```python
from build123d import *

# Parameters (mm, degrees)
IMPORTED_BODY_4_1_OUTLINE_W = 30
IMPORTED_BODY_4_1_OUTLINE_H = 14
IMPORTED_BODY_4_1_DEPTH     = 3
SKETCH_1_R                  = 3.5
SKETCH_1_R_2                = 2
SKETCH_1_R_3                = 6
CUT_EXTRUDE_1_DEPTH         = 3


# Read off the part's stored shape, not the designer's step: 基体零件-零件4-1
with BuildPart() as part:
    # 基体零件-零件4-1 outline → 基体零件-零件4-1 (new body)
    with BuildSketch(Plane.XY):
        Polygon((110, 31), (0, 31), (0, 20), (-3, 20), (-3, 10), (0, 10), (0, 0), (20, 0), (20, -3), (30, -3), (30, 0), (70, 0), (70, -3), (80, -3), (80, 0), (120, 0), (120, -3), (130, -3), (130, 0), (170, 0), (170, -3), (180, -3), (180, 0), (220, 0), (220, -3), (230, -3), (230, 0), (270, 0), (270, -3), (280, -3), (280, 0), (300, 0), (300, 10), (303, 10), (303, 20), (300, 20), (300, 31), (140, 31), (140, 23), (110, 23), align=None)
        with Locations((125, 13)):
            Rectangle(IMPORTED_BODY_4_1_OUTLINE_W, IMPORTED_BODY_4_1_OUTLINE_H, mode=Mode.SUBTRACT)
    extrude(amount=IMPORTED_BODY_4_1_DEPTH)

    # 草图1 → 切除-拉伸1 (cut)
    with BuildSketch(Plane(origin=(0, 0, 0), x_dir=(-1, 0, 0), z_dir=(0, 0, -1))):
        with Locations(Location((-147.5, 10, 0), (0, 0, 180))):
            Circle(SKETCH_1_R)
        with Locations(Location((-95, 3.5, 0), (0, 0, 180))):
            Circle(SKETCH_1_R_2)
        with Locations((-155.5, 27.5)):
            Circle(SKETCH_1_R_3)
    extrude(amount=-CUT_EXTRUDE_1_DEPTH, mode=Mode.SUBTRACT)


solid = part.part
```
Input: part model. Units: mm. Frame: model coordinates. Give positions to 0.01 mm unless a question says otherwise; leave off trailing zeros. Order: outer loops, then holes, each group sorted by start corner. A loop starts at its lowest first (then second) coordinate and runs counter-clockwise, first axis right, second up. Notation, with made-up numbers: M 88,88 L 135,88 A18 cw 135,110 Z; hole C 23.5,54 d5. An arc over 180 degrees is marked long. Return JSON: item names as keys, results as strings.
Item 1: Pull-direction query (X, two-part tool) for faces 1 (the flat face through (148, 14, 0)), 2 (the cylindrical face through (155.684, 21.503, 1.479)), 3 (the cylindrical face through (150.84, 8.95, 1.48)); classes: +X half, -X half, draft (parallel to the pull), parting line (faces both ways), or undercut.
Solutions:
{"face 1": "draft", "face 2": "undercut", "face 3": "undercut"}
Item 2: Cut plane B-B (y = 16.5). Return loops of the section in (x, z), then the cut area to 3 significant figures.
Solutions:
{"outline": "M -3,0 L 110,0 L 110,3 L -3,3 Z; M 140,0 L 303,0 L 303,3 L 140,3 Z", "area": "828 mm^2"}
Item 3: Cut plane C-C (z = 0.8). State how many separate pieces and enclosed holes the cut face has, then the cut area to 3 significant figures.
Solutions:
{"separate pieces": "1", "enclosed holes": "3", "area": "8,730 mm^2"}
Item 4: Cut plane D-D (x = 38.5). Return loops of the section in (y, z).
Solutions:
{"outline": "M 0,0 L 31,0 L 31,3 L 0,3 Z"}
Item 5: Cut plane A-A (x = 112.5). Return loops of the section in (y, z), then the cut area to 3 significant figures.
Solutions:
{"outline": "M 0,0 L 6,0 L 6,3 L 0,3 Z; M 20,0 L 23,0 L 23,3 L 20,3 Z", "area": "27.0 mm^2"}
Item 6: Ray query, probe 1 along X at (y, z) = (10.5, 2.3); probe 2 along X at (y, z) = (18, 1.35); probe 3 along X at (y, z) = (27.5, 0.7). Return the intervals inside material, ascending.
Solutions:
{"probe 1": "-3 to 110, 140 to 144.04, 150.96 to 303", "probe 2": "-3 to 110, 140 to 303", "probe 3": "0 to 110, 140 to 149.5, 161.5 to 300"}
Item 7: First-contact query: P1, Ø1, axis at y = 26.5, z = 2.5, coming from the -X side; P2, Ø1.5, axis at x = 6.5, z = 1.5, coming from the -Y side. Flat tips, straight axial feed; report the tip coordinate or a pass-through.
Solutions:
{"P1": "x = 0", "P2": "y = 0"}
